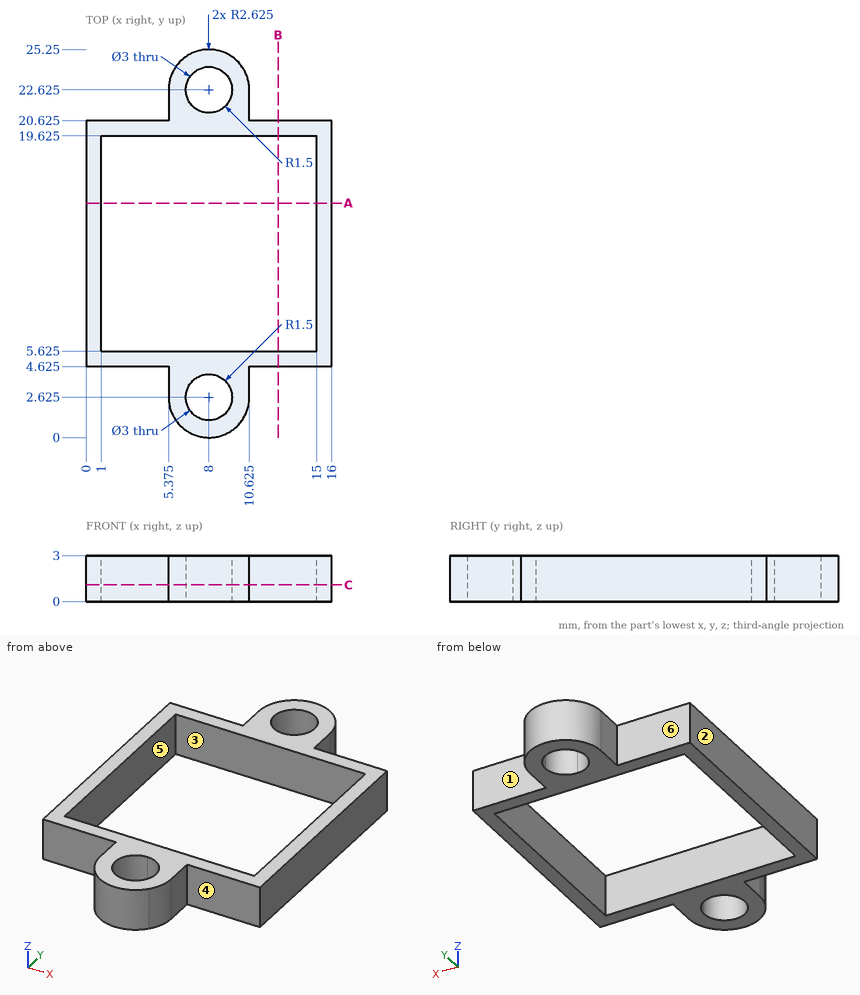
Can you work these out from the drawing? Everything is in mm from the part's minimum corner. A direction names the side the tool comes from. Coordinates: 2 decimals unless noted, no trailing zeros. Loops run counter-clockwise (first coordinate to the right, second up) from the corner with the lowest first, then second, coordinate; pieces in that order, holes last.
1) Imagine slicing it at C-C on z = 1.1. List the corners of the cut face in (x, y) for me (3 decimals).
2) For pin 1 (4 mm diameter, centred on x = 12, y = 6, fed in from -Z); pin 2 (1.5 mm diameter, centred on x = 3.5, z = 1, fed in from +Y) (3 decimals); pin 3 (1.5 mm diameter, centred on x = 1.5, z = 1, fed in from -Y) (3 decimals); pin 4 (1.8 mm diameter, centred on x = 8, y = 2.625, fed in from -Z), each with a flat end and sliding along its axis, tell me the tip position at first contact or that it passes through.
3) Thinking about a two-plate mould opening in X: for the marked faces 1, 2 and 3, which applies, pulls with the +X half, pulls with the -X half, needs draft (parallel to the pull), parting line crosses it, or undercut?
4) Imagine slicing it at B-B on x = 12.5. List the corners of the cut face in (y, z) for me (3 decimals), plus the area to 3 significant figures.
5) Which directions (+Z, -Z, +X, -X, +Y, -Y) give clear straight access to the entire face, cutting with the end or side of a thin tool? Please do the marked faces 4, 5 and 6.
6) Imagine slicing it at A-A on y = 15.25. List the corners of the cut face in (x, z) for me, plus the area to 3 significant figures.
7) I need wall thicknesses on probe 1 along Y at (x, z) = (8, 1.6) (3 decimals); probe 2 along Y at (x, z) = (1.5, 0.2) (3 decimals); probe 3 along X at (y, z) = (11.75, 0.5). Which ranges of each line are inside material? Lowest first, please.
Completed:
1. outline: (0, 4.625) - (5.375, 4.625) - (5.375, 2.625) arc R2.625 ccw to (10.625, 2.625) - (10.625, 4.625) - (16, 4.625) - (16, 20.625) - (10.625, 20.625) - (10.625, 22.625) arc R2.625 ccw to (5.375, 22.625) - (5.375, 20.625) - (0, 20.625) - close; hole (1, 5.625) - (15, 5.625) - (15, 19.625) - (1, 19.625) - close; hole circle Ø3 at (8, 2.625); hole circle Ø3 at (8, 22.625)
2. pin 1: stops at z = 0
2. pin 2: stops at y = 20.625
2. pin 3: stops at y = 4.625
2. pin 4: passes through
3. face 1: needs draft
3. face 2: pulls with the -X half
3. face 3: undercut
4. outline: (4.625, 0) - (5.625, 0) - (5.625, 3) - (4.625, 3) - close; (19.625, 0) - (20.625, 0) - (20.625, 3) - (19.625, 3) - close
4. area: 6.00 mm2
5. face 4: +Z, -Z, +X, -Y
5. face 5: +Z, -Z
5. face 6: +Z, -Z, -X, +Y
6. outline: (0, 0) - (1, 0) - (1, 3) - (0, 3) - close; (15, 0) - (16, 0) - (16, 3) - (15, 3) - close
6. area: 6.00 mm2
7. probe 1: y = 0 to 1.125, 4.125 to 5.625, 19.625 to 21.125, 24.125 to 25.25
7. probe 2: y = 4.625 to 5.625, 19.625 to 20.625
7. probe 3: x = 0 to 1, 15 to 16
